Geometry check sheet. Reference: the model listing, model coordinates, mm. A direction names the side the tool comes from. Round coordinates to 2 decimals unless told otherwise and drop trailing zeros. Write each loop counter-clockwise with the first axis right and the second up, starting at its lowest first coordinate (ties: lowest second). Pieces come first, ordered by that corner, then holes. Notation, with made-up numbers: (24, 46) - (82, 46) arc R29 ccw to (82, 66) - close; hole circle Ø8 at (34.5, -9). An arc over 180 degrees is marked (long way). Return JSON: item names as keys, results as strings. Group by question number.
from build123d import *

# Parameters (mm, degrees)
BOSS_EXTRUDE1_DEPTH            = 16
CBORE_FOR_M4_SHCS1_D           = 4.5
CBORE_FOR_M4_SHCS1_CBORE_D     = 8
CBORE_FOR_M4_SHCS1_CBORE_DEPTH = 4


with BuildPart() as part:
    # Sketch2 → Boss-Extrude1 (new body)
    with BuildSketch(Plane.XY):
        with BuildLine():
            Line((-49.5, 0.125), (-25.999699517, 0.125))
            ThreePointArc((-25.999699517, 0.125), (0, 26), (25.999699517, 0.125))
            Line((25.999699517, 0.125), (49.5, 0.125))
            Line((49.5, 0.125), (49.5, 10.125))
            Line((49.5, 10.125), (34.546843199, 10.125))
            ThreePointArc((34.546843199, 10.125), (0, 36), (-34.546843199, 10.125))
            Line((-34.546843199, 10.125), (-49.5, 10.125))
            Line((-49.5, 10.125), (-49.5, 0.125))
        make_face()
    extrude(amount=-BOSS_EXTRUDE1_DEPTH)

    # CBORE for M4 SHCS1 (through all)
    with Locations(Plane(origin=(0, 10.125, 0), x_dir=(1, 0, 0), z_dir=(0, 1, 0))):
        with Locations((-42.023421599, 8), (42.023421599, 8)):
            CounterBoreHole(CBORE_FOR_M4_SHCS1_D / 2, CBORE_FOR_M4_SHCS1_CBORE_D / 2, CBORE_FOR_M4_SHCS1_CBORE_DEPTH)


solid = part.part
1. Mould release check, pull along Z, two halves, no side actions. Record for faces 1 (the face through (39.88, 3.08, -8.68)), 2 (the face through (-4, 26, 0)), 3 (the face through (-40, 10.125, -4)), 4 (the face through (-4, 26, -16)): pulls with the +Z half, pulls with the -Z half, needs draft (parallel to the pull), parting line crosses it, or undercut.
2. Material ranges on line 1 along Y through (x, z) = (36.5, -8) (3 decimals); line 2 along Z through (x, y) = (-40, 9.5); line 3 along Y through (x, z) = (-18, -9.75), recorded low to high.
3. Depth check by flat-ended pin: pin 1 Ø6.5 at (x, z) = (41.5, -7) entering from +Y (3 decimals); pin 2 Ø10 at (x, y) = (-16, 31.5) entering from +Z; pin 3 Ø1.5 at (y, z) = (21.5, -4) entering from +X; pin 4 Ø6.5 at (x, z) = (-42.02, -8) entering from +Y (3 decimals). Enter the tip coordinate at first touch or a pass-through.
4. Tool access check on faces 5 (the face through (38.027, 8.153, -8.176)), 6 (the face through (44, 10.125, -4)), 7 (the face through (0.648, 35.994, -7.888)). Record the directions out of +Z, -Z, +X, -X, +Y, -Y that give a thin tool (end or side, any length) a straight path to the whole face; none if there is none.
5. Section check D-D (y = 27). Enter the section's corners in (x, z), and give its area (3 significant figures).
6. Section check C-C (x = 21). Enter the section's corners in (y, z), and give its area (3 significant figures).
Result sheet:
{
 "1": {"face 1": "undercut", "face 2": "pulls with the +Z half", "face 3": "needs draft", "face 4": "pulls with the -Z half"},
 "2": {"line 1": "y = 0.125 to 10.125", "line 2": "z = -16 to -11.45, -4.55 to 0", "line 3": "y = 18.76 to 31.18"},
 "3": {"pin 1": "stops at y = 10.125", "pin 2": "stops at z = 0", "pin 3": "stops at x = 29.42", "pin 4": "stops at y = 6.125"},
 "4": {"face 5": "+Y", "face 6": "+Z, -Z, +X, +Y", "face 7": "+Z, -Z, +Y"},
 "5": {"outline": "(-23.81, -16) - (23.81, -16) - (23.81, 0) - (-23.81, 0) - close", "area": "762 mm²"},
 "6": {"outline": "(15.33, -16) - (29.24, -16) - (29.24, 0) - (15.33, 0) - close", "area": "223 mm²"}
}
